Work out the finished part from the listing and answer in its coordinate system (mm). Face numbers are marked on the shaded views. A direction names the side the tool comes from. Round coordinates to 2 decimals unless told otherwise and drop trailing zeros. Write each loop counter-clockwise with the first axis right and the second up, starting at its lowest first coordinate (ties: lowest second). Pieces come first, ordered by that corner, then holes. Notation, with made-up numbers: (89.5, 23.25) -> (137.5, 23.25) arc R29 ccw to (137.5, 46.25) -> close; hole circle Ø7 at (-5, -22.5). An arc over 180 degrees is marked (long way). One line per question, with ' | ' between items. Start each with the question number.
```python
from build123d import *

# Parameters (mm, degrees)
F1_DEPTH = 25.4
F3_DEPTH = 12.7
F4_W     = 17.007686
F4_H     = 13.244051
F5_DEPTH = 25.4
F7_DEPTH = 25.4


with BuildPart() as f1:
    # F0 (on Front) → F1 (new body)
    with BuildSketch(Plane.XZ):
        with BuildLine():
            Line((-11.337823, 21.661693), (-11.337823, 35.488307))
            ThreePointArc((-11.337823, 35.488307), (-35.166102, 44.785234), (-58.532663, 34.382179))
            Line((-58.532663, 34.382179), (-58.532663, 21.661693))
            Line((-58.532663, 21.661693), (-48.20931, 21.661693))
            Line((-48.20931, 21.661693), (-48.20931, 3.963629))
            Line((-48.20931, 3.963629), (-11.337823, 3.963629))
            Line((-11.337823, 3.963629), (-11.337823, 21.661693))
        make_face()
    extrude(amount=F1_DEPTH)

    # F2 (on face) → F3 (join)
    with BuildSketch(Plane(origin=(0, 0, 3.963629), x_dir=(1, 0, 0), z_dir=(0, 0, -1))):
        Polygon((-11.337823, -70.18809), (-11.337823, 0), (-48.20931, 0), (-65.216996, 0), (-65.216996, -70.18809), align=None)
    extrude(amount=-F3_DEPTH)

    # F4 (on face) → F5 (cut)
    with BuildSketch(Plane.XY.offset(16.663629)):
        with Locations((-56.713153, 6.622025)):
            Rectangle(F4_W, F4_H)
    extrude(amount=-F5_DEPTH, mode=Mode.SUBTRACT)

    # F6 (on face) → F7 (cut)
    with BuildSketch(Plane.XY.offset(16.663629)):
        with BuildLine():
            Line((-53.567118, 70.18809), (-50.555244, 43.886501))
            ThreePointArc((-50.555244, 43.886501), (-40.800313, 36.453912), (-33.769552, 46.502318))
            Line((-33.769552, 46.502318), (-38.451883, 70.18809))
            Line((-38.451883, 70.18809), (-53.567118, 70.18809))
        make_face()
    extrude(amount=-F7_DEPTH, mode=Mode.SUBTRACT)


solid = f1.part
```
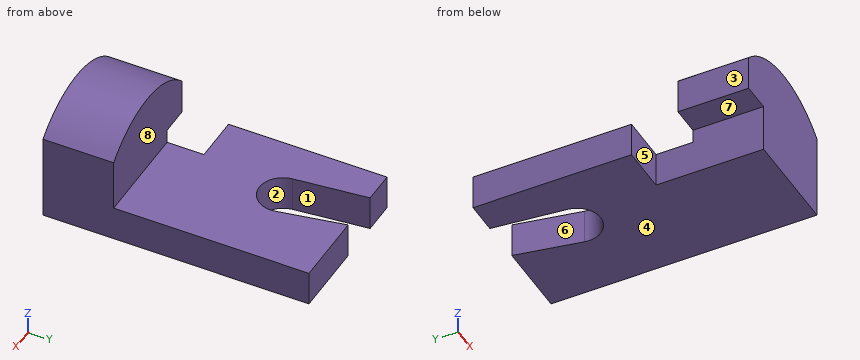
(1) Consider L1, parallel to X at y = -1, z = 6; L2, parallel to X at y = 64.5, z = 13; L3, parallel to Z at x = -57.5, y = 35. Determine where each line is inside the solid, lowest interval first.
(2) A cutting plane is placed at B-B, the plane z = 11. Determine the outline of the cut face in (x, y).
(3) A cutting plane is placed at A-A, the plane y = 38. Determine the outline of the cut face in (x, z).
(4) A cutting plane is placed at D-D, the plane y = -15. Determine the outline of the cut face in (x, z).
(5) For the marked faces 5, 6, 7 and 8, determine the directions among +Z, -Z, +X, -X, +Y, -Y from which every point of the face is accessible in a straight line to the end or side of a thin tool.
(6) A cutting plane is placed at C-C, the plane x = -55.5. Determine the outline of the cut face in (y, z), then the cut area to 3 significant figures.
(7) The mould has two halves that part along X. Classify the marked faces 1, 2, 3 and 4: +X half, -X half, draft (parallel to the pull), parting line (faces both ways), or undercut.
(8) Given pin 1 Ø8 at (x, z) = (-49.5, 23) entering from +Y; pin 2 Ø14 at (y, z) = (-7, 8.5) entering from -X; pin 3 Ø4 at (y, z) = (-12.5, 29.5) entering from -X, each flat-ended and moving along its own axis, determine where each tip first touches the part or whether it passes through.
Returned:
1) L1: -48.21 to -11.34 | L2: -65.22 to -52.92, -37.33 to -11.34 | L3: 3.96 to 16.66
2) outline: (-65.22, 13.24) -> (-48.21, 13.24) -> (-48.21, -25.4) -> (-11.34, -25.4) -> (-11.34, 70.19) -> (-38.45, 70.19) -> (-33.77, 46.5) arc R8.5 cw (long way) to (-50.56, 43.89) -> (-53.57, 70.19) -> (-65.22, 70.19) -> close
3) outline: (-65.22, 3.96) -> (-47.14, 3.96) -> (-47.14, 16.66) -> (-65.22, 16.66) -> close; (-37.08, 3.96) -> (-11.34, 3.96) -> (-11.34, 16.66) -> (-37.08, 16.66) -> close
4) outline: (-58.53, 21.66) -> (-48.21, 21.66) -> (-48.21, 3.96) -> (-11.34, 3.96) -> (-11.34, 35.49) arc R33.2 ccw to (-58.53, 34.38) -> close
5) face 5: +Z, -Z, -X, -Y | face 6: +Z, -Z | face 7: -Z, -X, +Y, -Y | face 8: +Z, +X, -X, +Y
6) outline: (-25.4, 21.66) -> (0, 21.66) -> (0, 37.22) -> (-25.4, 37.22) -> close; (13.24, 3.96) -> (70.19, 3.96) -> (70.19, 16.66) -> (13.24, 16.66) -> close | area: 1,120 mm2
7) face 1: undercut | face 2: undercut | face 3: -X half | face 4: draft
8) pin 1: y = 0 | pin 2: x = -48.21 | pin 3: x = -58.53
